from build123d import *

# Parameters (mm, degrees)
RESSALTO_EXTRUS_O1_DEPTH = 3
ESBO_O2_R                = 1.5
CORTE_EXTRUS_O1_DEPTH    = 10
ESBO_O3_W                = 3
ESBO_O3_H                = 25
CORTE_EXTRUS_O2_DEPTH    = 10


with BuildPart() as part:
    # Esboço1 → Ressalto-extrusão1 (new body)
    with BuildSketch(Plane.XY):
        with BuildLine():
            Line((43.040081042, -11.381695114), (56.040081042, -11.381695114))
            Line((56.040081042, -11.381695114), (56.040081042, 28.618304886))
            ThreePointArc((56.040081042, 28.618304886), (50.182216666, 42.76044051), (36.040081042, 48.618304886))
            Line((36.040081042, 48.618304886), (-16.959918958, 48.618304886))
            ThreePointArc((-16.959918958, 48.618304886), (-31.102054581, 42.76044051), (-36.959918958, 28.618304886))
            Line((-36.959918958, 28.618304886), (-36.959918958, -1.381695114))
            Line((-36.959918958, -1.381695114), (-36.959918958, -16.381695114))
            Line((-36.959918958, -16.381695114), (-11.959918958, -16.381695114))
            Line((-11.959918958, -16.381695114), (-11.959918958, -11.381695114))
            Line((-11.959918958, -11.381695114), (18.040081042, -11.381695114))
            Line((18.040081042, -11.381695114), (18.040081042, -16.381695114))
            Line((18.040081042, -16.381695114), (43.040081042, -16.381695114))
            Line((43.040081042, -16.381695114), (43.040081042, -11.381695114))
        make_face()
    extrude(amount=RESSALTO_EXTRUS_O1_DEPTH)

    # Esboço2 → Corte-extrusão1 (cut)
    with BuildSketch(Plane(origin=(0, 0, 0), x_dir=(-1, 0, 0), z_dir=(0, 0, -1))):
        with Locations((21.959918958, 35.668304886)):
            Circle(ESBO_O2_R)
        with Locations((21.959918958, -6.381695114)):
            Circle(ESBO_O2_R)
    extrude(amount=-CORTE_EXTRUS_O1_DEPTH, mode=Mode.SUBTRACT)

    # Esboço3 → Corte-extrusão2 (cut)
    with BuildSketch(Plane.XY.offset(3)):
        with Locations((-3.459918958, 21.118304886)):
            Rectangle(ESBO_O3_W, ESBO_O3_H)
        with Locations((44.540081042, 21.118304886)):
            Rectangle(ESBO_O3_W, ESBO_O3_H)
    extrude(amount=-CORTE_EXTRUS_O2_DEPTH, mode=Mode.SUBTRACT)


solid = part.part
Could you check a few things on this model? Use its own coordinates, in mm. A direction names the side the tool comes from. Give positions to 0.01 mm unless a question says otherwise; leave off trailing zeros. Order: outer loops, then holes, each group sorted by start corner. A loop starts at its lowest first (then second) coordinate and runs counter-clockwise, first axis right, second up.
1. We'd pull the mould along Y, two halves only. Please class faces 1 (the cylindrical face through (-23.39, -5.93, 1.48)), 2 (the flat face through (30, -16.382, 1)), 3 (the flat face through (43.04, -14, 1)): pulls with the +Y half, pulls with the -Y half, needs draft (parallel to the pull), parting line crosses it, or undercut.
2. Suppose I cut it at A-A (y = 18.5). List the corners of the cut face in (x, z) for me.
3. Suppose I cut it at C-C (x = 16). List the corners of the cut face in (y, z) for me.
4. I need wall thicknesses on L1, parallel to X at y = 21.5, z = 1.85; L2, parallel to Y at x = -4, z = 0.7; L3, parallel to X at y = 31, z = 2.3. Which ranges of each line are inside material? Lowest first, please.
5. For faces 4 (the flat face through (-11.96, -14, 1)), 5 (the flat face through (49, -11.382, 1)), 6 (the flat face through (46.04, 21, 2)), which set-ups out of +Z, -Z, +X, -X, +Y, -Y let a thin tool reach every point of the face, with its end or its side?
6. Will these pins go through, and if not, where does the flat tip stop? P1, Ø0.9, axis at x = -4, z = 1, coming from the -Y side; P2, Ø0.9, axis at y = -13.5, z = 1, coming from the +X side; P3, Ø1, axis at y = 40.5, z = 1, coming from the +X side; P4, Ø2.5, axis at x = -21.96, y = -6.38, coming from the -Z side.
7. Suppose I cut it at B-B (z = 0.45). List the corners of the cut face in (x, y) for me.
8. Suppose I cut it at D-D (y = 44). List the corners of the cut face in (x, z) for me.
Solved:
1. face 1: undercut
1. face 2: pulls with the -Y half
1. face 3: needs draft
2. outline: (-36.96, 0) - (-4.96, 0) - (-4.96, 3) - (-36.96, 3) - close; (-1.96, 0) - (43.04, 0) - (43.04, 3) - (-1.96, 3) - close; (46.04, 0) - (56.04, 0) - (56.04, 3) - (46.04, 3) - close
3. outline: (-11.38, 0) - (48.62, 0) - (48.62, 3) - (-11.38, 3) - close
4. L1: x = -36.96 to -4.96, -1.96 to 43.04, 46.04 to 56.04
4. L2: y = -11.38 to 8.62, 33.62 to 48.62
4. L3: x = -36.82 to -4.96, -1.96 to 43.04, 46.04 to 55.9
5. face 4: +Z, -Z, -Y
5. face 5: +Z, -Z, +X, -Y
5. face 6: +Z, -Z
6. P1: stops at y = -11.38
6. P2: stops at x = 43.04
6. P3: stops at x = 52.49
6. P4: passes through
7. outline: (-36.96, -16.38) - (-11.96, -16.38) - (-11.96, -11.38) - (18.04, -11.38) - (18.04, -16.38) - (43.04, -16.38) - (43.04, -11.38) - (56.04, -11.38) - (56.04, 28.62) arc R20 ccw to (36.04, 48.62) - (-16.96, 48.62) arc R20 ccw to (-36.96, 28.62) - close; hole circle Ø3 at (-21.96, -6.38); hole circle Ø3 at (-21.96, 35.67); hole (-4.96, 8.62) - (-1.96, 8.62) - (-1.96, 33.62) - (-4.96, 33.62) - close; hole (43.04, 8.62) - (46.04, 8.62) - (46.04, 33.62) - (43.04, 33.62) - close
8. outline: (-29.74, 0) - (48.82, 0) - (48.82, 3) - (-29.74, 3) - close
